The figure shows three views and two pictorial views of one solid part (mm, origin at its lowest corner). Answer the questions. A direction names the side the tool comes from. Coordinates: 2 decimals unless noted, no trailing zeros. Order: outer loops, then holes, each group sorted by start corner. A loop starts at its lowest first (then second) coordinate and runs counter-clockwise, first axis right, second up. Notation, with made-up numbers: (-6, 84) - (44, 84) arc R34 ccw to (44, 120) - close; hole circle Ø5 at (6, 22.25). An arc over 180 degrees is marked (long way). Use one line per item in the form item = value. Start each with the question number.
Item 1: Consider line 1 along Z through (x, y) = (25, 2.1); line 2 along Z through (x, y) = (5, 2.95); line 3 along X through (y, z) = (3.2, 18.5) (1 decimal). Determine where each line is inside the solid, lowest interval first. Write a range as [from, to].
Item 2: Section B-B, the plane z = 15 is taken. Write down the section's boundary in (x, y), and give its area (3 significant figures).
Item 3: Section A-A, the plane x = 25 is taken. Write down the section's boundary in (y, z), and give its area (3 significant figures).
Item 4: Section C-C, the plane y = 3.5 is taken. Write down the section's boundary in (x, z).
Item 5: Each of these flat-tipped pins is pushed along its axis until it touches: pin 1 Ø13 at (x, z) = (25, 12) entering from +Y (1 decimal); pin 2 Ø3 at (y, z) = (3, 16) entering from -X. Where does it stop, or does it pass through?
Item 6: The mould has two halves that part along Z. Classify the marked faces 3, 4 and 5: released by +Z, released by -Z, zero draft, split by the parting line, or undercut.
Item 7: A tool of negligible diameter and unlimited length cuts with its end or side. For the marked faces 1 and 2, from which of +Z, -Z, +X, -X, +Y, -Y can it reach the whole face along a straight path? Write none if from no direction.
Item 8: Section D-D, the plane z = 21.25 is taken. Write down the section's boundary in (x, y).
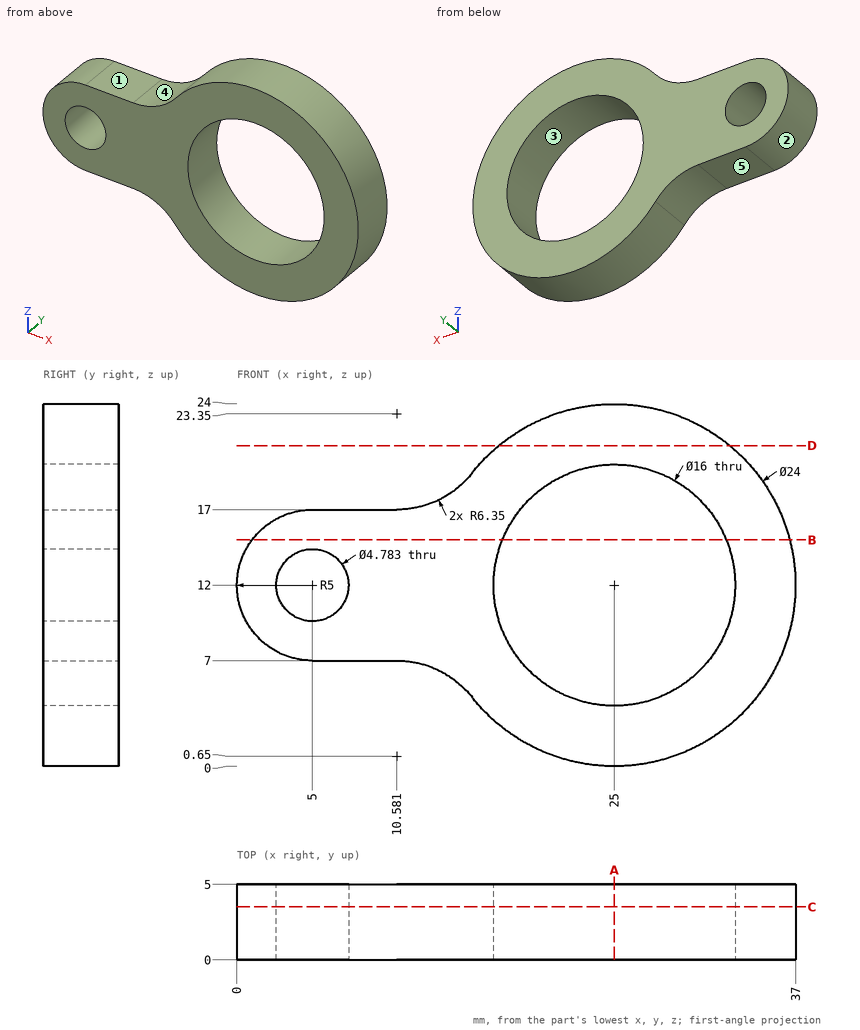
Response:
q1.line_1 = [0, 4], [20, 24]
q1.line_2 = [7, 9.61], [14.39, 17]
q1.line_3 = [14.7, 20.3], [29.7, 35.1]
q2.outline = (1, 0) - (17.58, 0) - (17.58, 5) - (1, 5) - close; (32.42, 0) - (36.62, 0) - (36.62, 5) - (32.42, 5) - close
q2.area = 104 mm2
q3.outline = (0, 0) - (5, 0) - (5, 4) - (0, 4) - close; (0, 20) - (5, 20) - (5, 24) - (0, 24) - close
q3.area = 40.0 mm2
q4.outline = (5, 7) - (10.58, 7) arc R6.35 cw to (15.57, 4.58) arc R12 ccw (long way) to (15.57, 19.42) arc R6.35 cw to (10.58, 17) - (5, 17) arc R5 ccw to start; hole circle Ø4.78 at (5, 12); hole circle Ø16 at (25, 12)
q5.pin_1 = through
q5.pin_2 = 0.67
q6.face_3 = undercut
q6.face_4 = released by +Z
q6.face_5 = released by -Z
q7.face_1 = +Z, -X, +Y, -Y
q7.face_2 = -X, +Y, -Y
q8.outline = (17.36, 0) - (32.64, 0) - (32.64, 5) - (17.36, 5) - close
